Work out the finished part from the listing and answer in its coordinate system (mm). Face numbers are marked on the shaded views. A direction names the side the tool comes from. Round coordinates to 2 decimals unless told otherwise and drop trailing zeros. Loops run counter-clockwise (first coordinate to the right, second up) from the corner with the lowest first, then second, coordinate; pieces in that order, holes last. Notation, with made-up numbers: M -0.5,-39.5 L 54.5,-39.5 A13 ccw 54.5,-28.5 Z; hole C 40,89.25 d4. An arc over 180 degrees is marked long. One line per item, written item: value.
Autodesk Inventor part; units mm, degrees
ref_plane "YZ Plane" through (0, 0, 0) normal (1, 0, 0) x (0, 1, 0)
ref_plane "XZ Plane" through (0, 0, 0) normal (0, 1, 0) x (-1, 0, 0)
ref_plane "XY Plane" through (0, 0, 0) normal (0, 0, 1) x (1, 0, 0)
sketch "Sketch1" plane through (0, 0, 0) normal (1, 0, 0) x (0, 1, 0)
  circle A0 centre (0, 0) radius 6.096
  dimension "d0" = 12.192
extrude "Extrusion1" add sketch "Sketch1" along normal blind 127.7874
sketch "Sketch2" plane through (0, 0, 0) normal (-1, 0, 0) x (0, 0, 1)
  circle A0 centre (0, 0) radius 3.175
  circle A1 centre (0, 0) radius 3.175
  dimension "d3" = 6.35
extrude "Extrusion2" add sketch "Sketch2" along normal blind 12.7
sketch "Sketch3" plane through (127.7874, 0, 0) normal (1, 0, 0) x (0, 0, -1)
  circle A0 centre (0, 0) radius 3.81
  dimension "d6" = 7.62
extrude "Extrusion3" add sketch "Sketch3" along normal blind 12.7
properties part number "conveyor roller"
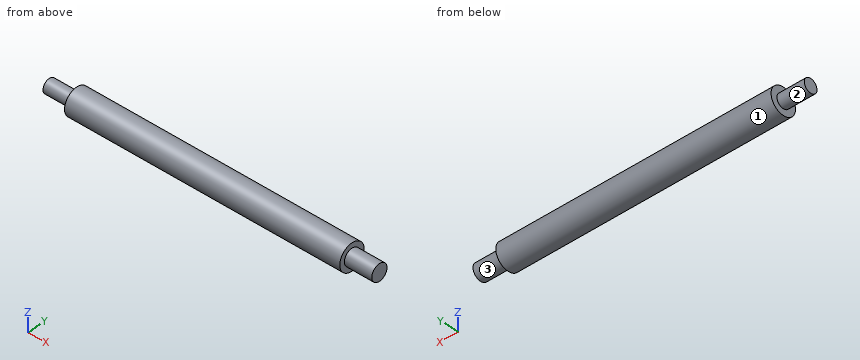
1) Find the intervals of material crossed by probe 1 along X at (y, z) = (5, 1); probe 2 along X at (y, z) = (3.25, -1.25); probe 3 along Y at (x, z) = (129.5, -2.25), in increasing order. Write a range as from..to.
Check values:
probe 1: 0..127.79
probe 2: 0..140.49
probe 3: -3.07..3.07
2) Each of these flat-tipped pins is pushed along its axis until it touches: pin 1 (1 mm diameter, centred on x = 71, z = -4.5, fed in from -Y); pin 2 (2 mm diameter, centred on x = 4.5, z = 3, fed in from +Y); pin 3 (1.5 mm diameter, centred on x = 109.5, y = 5, fed in from +Z). Where does it stop, or does it pass through?
Check values:
pin 1: y = -4.6
pin 2: y = 5.76
pin 3: z = 4.37
3) Find section C-C (x = 79.5). Give the vertices of the cut face in (y, z), then the cut area to 3 significant figures.
Check values:
outline: C 0,0 d12.19
area: 117 mm2
4) Find section A-A (y = 0). Give the vertices of the cut face in (x, z) (3 decimals), then the cut area to 3 significant figures.
Check values:
outline: M -12.7,-3.175 L 0,-3.175 L 0,-6.096 L 127.787,-6.096 L 127.787,-3.81 L 140.487,-3.81 L 140.487,3.81 L 127.787,3.81 L 127.787,6.096 L 0,6.096 L 0,3.175 L -12.7,3.175 Z
area: 1,740 mm2
5) For the marked faces 1, 2 and 3, determine the directions among +Z, -Z, +X, -X, +Y, -Y from which every point of the face is accessible in a straight line to the end or side of a thin tool.
Check values:
face 1: +X, -X
face 2: -X
face 3: +X
